The drawing under review shows one solid part. Ordinate dimensions are in mm from its lowest x, y, z. A direction names the side the tool comes from. Give positions to 0.01 mm unless a question says otherwise; leave off trailing zeros. Order: outer loops, then holes, each group sorted by start corner. A loop starts at its lowest first (then second) coordinate and runs counter-clockwise, first axis right, second up. Notation, with made-up numbers: (-27, 80) -> (-2, 80) arc R13 cw to (-2, 101) -> close; hole circle Ø2 at (32.25, 15.5). An arc over 180 degrees is marked (long way). One line per item, written item: value. Start each with the question number.
1) Wall thickness on line 1 along X through (y, z) = (5.9, 35); line 2 along X through (y, z) = (22.75, 34); line 3 along Y through (x, z) = (6, 37.5): over which ranges is each line inside the solid? List them lowest first. Write a range as from..to.
2) Consider section B-B (x = 44.5). State the section outline as (y, z) points, plus the area to 3 significant figures.
3) Tool access review of the marked faces 4 and 5: name each direction out of +Z, -Z, +X, -X, +Y, -Y from which nothing blocks a thin tool from reaching the whole face with its end or side.
4) The part is to be moulded in two halves that separate along X. For the marked faces 1, 2 and 3, say which applies: released by +X, released by -X, zero draft, split by the parting line, or undercut.
5) Consider section A-A (y = 19.25). State the section outline as (x, z) points.
6) For pin 1 (5 mm diameter, centred on x = 23.5, z = 35, fed in from +Y); pin 2 (6.5 mm diameter, centred on x = 55.5, z = 52, fed in from +Y); pin 3 (2.5 mm diameter, centred on x = 65.5, z = 35, fed in from -Y), all flat-tipped, find the tip position at first contact; note any pin that passes through.
7) Consider section D-D (z = 77). State the section outline as (x, y) points.
8) Consider section C-C (x = 34). State the section outline as (y, z) points.
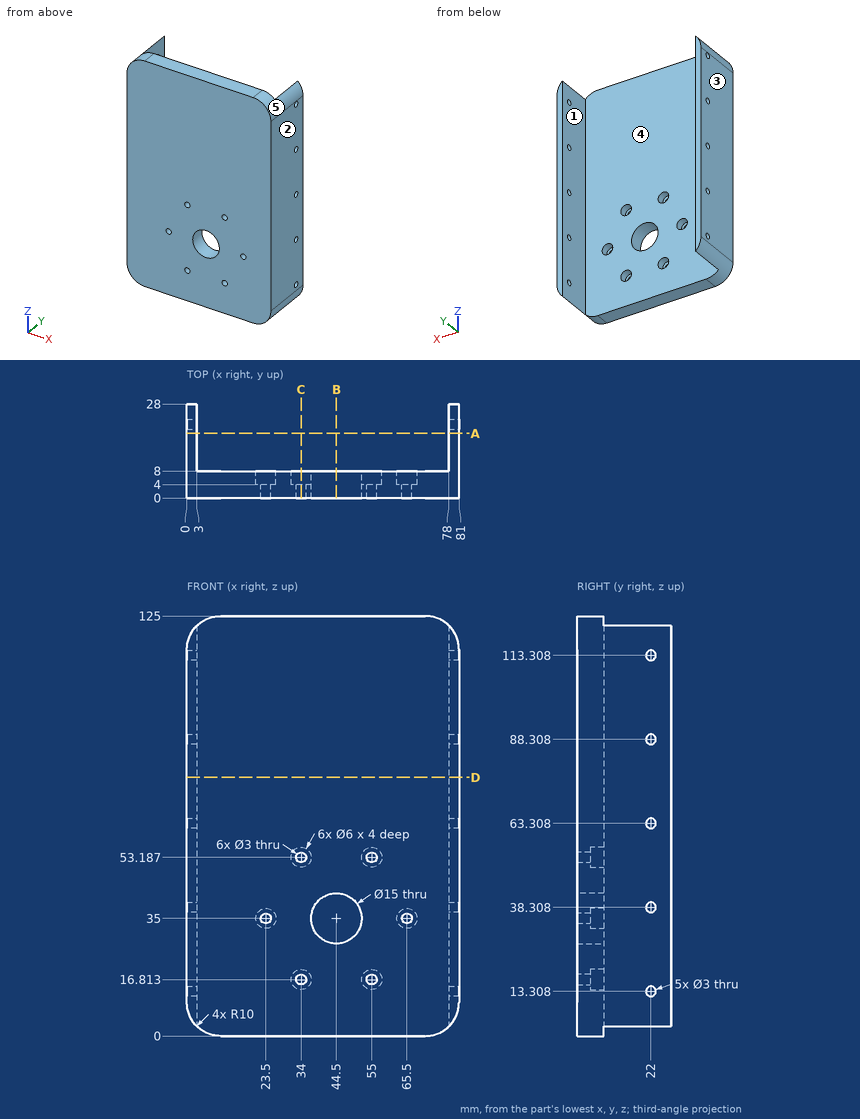
Checked values:
1. line 1: x = 0..20.5, 26.5..37, 52..62.5, 68.5..81
1. line 2: x = 0..3, 78..81
1. line 3: y = 0..8
2. outline: (0, 0) -> (8, 0) -> (8, 27.5) -> (0, 27.5) -> close; (0, 42.5) -> (8, 42.5) -> (8, 125) -> (0, 125) -> close
2. area: 880 mm^2
3. face 4: +Z, -Z, +Y
3. face 5: +Z, +X, +Y, -Y
4. face 1: undercut
4. face 2: released by +X
4. face 3: released by -X
5. outline: (0, 10) arc R10 ccw to (3, 2.86) -> (3, 122.14) arc R10 ccw to (0, 115) -> close; (78, 2.86) arc R10 ccw to (81, 10) -> (81, 115) arc R10 ccw to (78, 122.14) -> close
6. pin 1: stops at y = 4
6. pin 2: stops at y = 8
6. pin 3: passes through
7. outline: (0, 0) -> (81, 0) -> (81, 28) -> (78, 28) -> (78, 8) -> (3, 8) -> (3, 28) -> (0, 28) -> close
8. outline: (0, 0) -> (8, 0) -> (8, 13.81) -> (4, 13.81) -> (4, 15.31) -> (0, 15.31) -> close; (0, 18.31) -> (4, 18.31) -> (4, 19.81) -> (8, 19.81) -> (8, 50.19) -> (4, 50.19) -> (4, 51.69) -> (0, 51.69) -> close; (0, 54.69) -> (4, 54.69) -> (4, 56.19) -> (8, 56.19) -> (8, 125) -> (0, 125) -> close
